Geometry: see drawing. Coordinates: mm, zero at the bounding-box minimum. Give positions to 0.01 mm unless a question says otherwise; leave off trailing zeros. Loops run counter-clockwise (first coordinate to the right, second up) from the corner with the lowest first, then second, coordinate; pieces in that order, holes last. Notation, with made-up numbers: (-1, 66) -> (35, 66) arc R27 ccw to (35, 84) -> close; hole circle Ø11 at (42, 0). An arc over 180 degrees is marked (long way). Return JSON: item names as keys, results as strings. Group by question number.
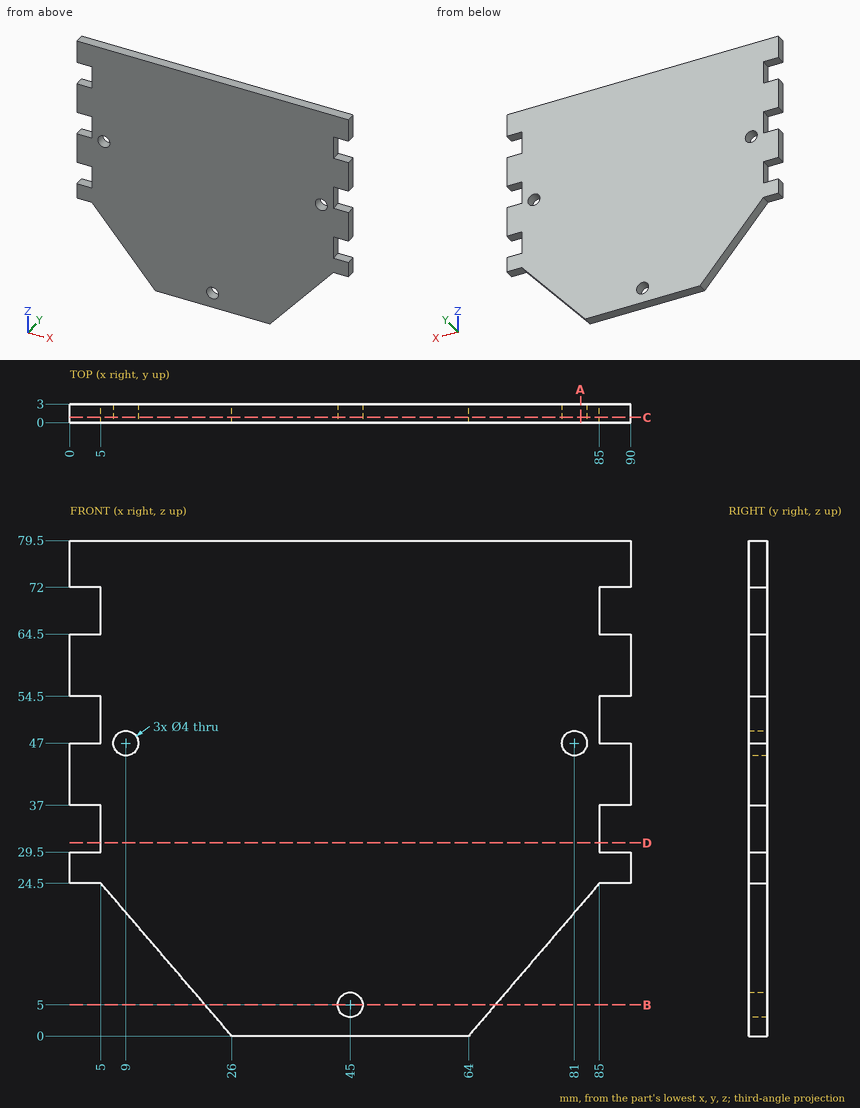
1) Cut plane D-D on z = 31. Return loops of the section in (x, y).
2) Material intervals for line 1 (Z direction, x = 85.5, y = 1.9); line 2 (X direction, y = 2.75, z = 33.5); line 3 (X direction, y = 0.75, z = 48.5), sorted ascending.
3) Cut plane C-C on y = 0.85. Count the separate pieces of the cut face and the enclosed holes in it, then the cut area to 3 significant figures.
4) Contact query for flat-ended pins moving along their axis: P1, Ø0.9, axis at y = 1.5, z = 52.5, coming from the -X side; P2, Ø1.5, axis at y = 1.5, z = 66.5, coming from the +X side; P3, Ø0.9, axis at x = 86.5, y = 1.5, coming from the -Z side. Output: stop coordinate, or through.
5) Cut plane A-A on x = 82. Return loops of the section in (y, z).
6) Cut plane B-B on z = 5. Return loops of the section in (x, y).
Calculated:
{
 "1": {"outline": "(5, 0) -> (85, 0) -> (85, 3) -> (5, 3) -> close"},
 "2": {"line 1": "24.5 to 29.5, 37 to 47, 54.5 to 64.5, 72 to 79.5", "line 2": "5 to 85", "line 3": "5 to 7.68, 10.32 to 79.68, 82.32 to 85"},
 "3": {"separate pieces": "1", "enclosed holes": "3", "area": "6,130 mm2"},
 "4": {"P1": "x = 5", "P2": "x = 85", "P3": "z = 24.5"},
 "5": {"outline": "(0, 21) -> (3, 21) -> (3, 45.27) -> (0, 45.27) -> close; (0, 48.73) -> (3, 48.73) -> (3, 79.5) -> (0, 79.5) -> close"},
 "6": {"outline": "(21.71, 0) -> (43, 0) -> (43, 3) -> (21.71, 3) -> close; (47, 0) -> (68.29, 0) -> (68.29, 3) -> (47, 3) -> close"}
}
